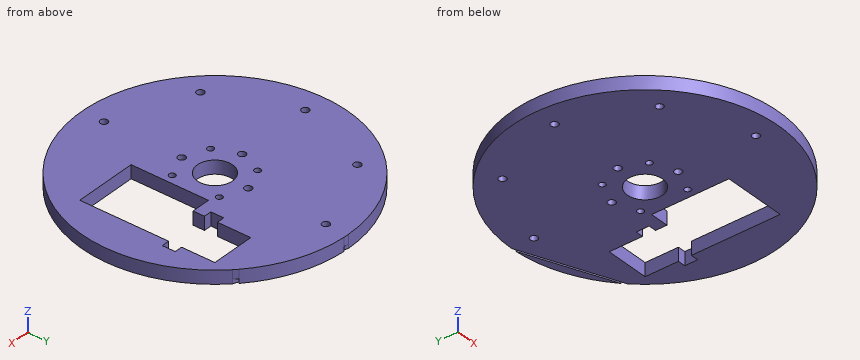
from build123d import *

# Parameters (mm, degrees)
SKETCH1_R              = 60
SKETCH1_R_2            = 8
SKETCH1_R_3            = 1.75
SKETCH1_R_4            = 1.5
BOSS_EXTRUDE1_DEPTH    = 6
CUT_EXTRUDE6_DEPTH     = 86.064681273
CUT_EXTRUDE7_DEPTH     = 2
MOVE_FACE2_OUTLINE_R   = 8
MOVE_FACE2_OUTLINE_R_2 = 7.92
MOVE_FACE2_OUTLINE_R_3 = 1.75
MOVE_FACE2_OUTLINE_R_4 = 1.67
MOVE_FACE2_OUTLINE_R_5 = 1.5
MOVE_FACE2_OUTLINE_R_6 = 1.42
MOVE_FACE2_DEPTH       = 6
MOVE_START             = 2
MOVE_FACE2_2_DEPTH     = 4


# Read off the part's stored shape, not the designer's step: Move Face2
with BuildPart() as part:
    # Sketch1 → Boss-Extrude1 (new body)
    with BuildSketch(Plane.XY):
        Circle(SKETCH1_R)
        Circle(SKETCH1_R_2, mode=Mode.SUBTRACT)
        with Locations((0, -15)):
            Circle(SKETCH1_R_3, mode=Mode.SUBTRACT)
        with Locations((10.606601718, -10.606601718)):
            Circle(SKETCH1_R_4, mode=Mode.SUBTRACT)
        with Locations((0, -50)):
            Circle(SKETCH1_R_3, mode=Mode.SUBTRACT)
        with Locations((-15, 0)):
            Circle(SKETCH1_R_3, mode=Mode.SUBTRACT)
        with Locations((-10.606601718, -10.606601718)):
            Circle(SKETCH1_R_4, mode=Mode.SUBTRACT)
        with Locations((0, 15)):
            Circle(SKETCH1_R_3, mode=Mode.SUBTRACT)
        with Locations((-10.606601718, 10.606601718)):
            Circle(SKETCH1_R_4, mode=Mode.SUBTRACT)
        with Locations((10.606601718, 10.606601718)):
            Circle(SKETCH1_R_4, mode=Mode.SUBTRACT)
        with Locations((-35.355339059, -35.355339059)):
            Circle(SKETCH1_R_3, mode=Mode.SUBTRACT)
        with Locations((-35.355339059, 35.355339059)):
            Circle(SKETCH1_R_3, mode=Mode.SUBTRACT)
        with Locations((-50, 0)):
            Circle(SKETCH1_R_3, mode=Mode.SUBTRACT)
        with Locations((0, 50)):
            Circle(SKETCH1_R_3, mode=Mode.SUBTRACT)
    extrude(amount=BOSS_EXTRUDE1_DEPTH)

    # Sketch7 → Cut-Extrude6 (cut, through all)
    with BuildSketch(Plane(origin=(0, 0, 0), x_dir=(-1, 0, 0), z_dir=(0, 0, -1))):
        Polygon((-43, -26), (-23, -26), (-14.5, -26), (-14.5, 9), (-23, 9), (-23, 14), (-19.5, 14), (-19.5, 20), (-23, 20), (-23, 35), (-43, 35), (-43, 20), (-46.5, 20), (-46.5, 14), (-43, 14), align=None)
    extrude(amount=-CUT_EXTRUDE6_DEPTH, mode=Mode.SUBTRACT)

    # Sketch8 → Cut-Extrude7 (cut)
    with BuildSketch(Plane(origin=(0, 0, 0), x_dir=(-1, 0, 0), z_dir=(0, 0, -1))):
        Polygon((-42.426406871, 42.426406871), (0, 60), (-0.316144007, 60.951441065), (-42.742550878, 43.377847936), align=None)
    extrude(amount=-CUT_EXTRUDE7_DEPTH, mode=Mode.SUBTRACT)

    # Move Face2 outline → Move Face2 (add)
    # profile 1 of 16: a face of its own
    with BuildSketch(Plane.XY):
        with BuildLine():
            ThreePointArc((0.01591808, 60.079997891), (-22.991620616, -55.506682313), (42.47171814, 42.494229705))
            Line((42.47171814, 42.494229705), (0.01591808, 60.079997891))
        make_face()
        with BuildLine():
            Line((0, 60), (42.426406871, 42.426406871))
            ThreePointArc((42.426406871, 42.426406871), (-22.961005942, -55.432771951), (0, 60))
        make_face(mode=Mode.SUBTRACT)
    # profile 2 of 16: a face of its own
    with BuildSketch(Plane.XY):
        with BuildLine():
            ThreePointArc((40.811514416, 44.091118052), (22.991620617, 55.506682313), (2.319029971, 60.035227159))
            Line((2.319029971, 60.035227159), (40.811514416, 44.091118052))
        make_face()
        with BuildLine():
            ThreePointArc((2.767270729, 59.936151134), (22.961005942, 55.432771951), (40.424503007, 44.338014803))
            Line((40.424503007, 44.338014803), (2.767270729, 59.936151134))
        make_face(mode=Mode.SUBTRACT)
    # profile 3 of 16: a face of its own
    with BuildSketch(Plane.XY):
        Circle(MOVE_FACE2_OUTLINE_R)
        Circle(MOVE_FACE2_OUTLINE_R_2, mode=Mode.SUBTRACT)
    # profile 4 of 16: a face of its own
    with BuildSketch(Plane.XY):
        with Locations((0, -15)):
            Circle(MOVE_FACE2_OUTLINE_R_3)
        with Locations((0, -15)):
            Circle(MOVE_FACE2_OUTLINE_R_4, mode=Mode.SUBTRACT)
    # profile 5 of 16: a face of its own
    with BuildSketch(Plane.XY):
        with Locations((10.606601718, -10.606601718)):
            Circle(MOVE_FACE2_OUTLINE_R_5)
        with Locations((10.606601718, -10.606601718)):
            Circle(MOVE_FACE2_OUTLINE_R_6, mode=Mode.SUBTRACT)
    # profile 6 of 16: a face of its own
    with BuildSketch(Plane.XY):
        with Locations((0, -50)):
            Circle(MOVE_FACE2_OUTLINE_R_3)
        with Locations((0, -50)):
            Circle(MOVE_FACE2_OUTLINE_R_4, mode=Mode.SUBTRACT)
    # profile 7 of 16: a face of its own
    with BuildSketch(Plane.XY):
        with Locations((-35.355339059, -35.355339059)):
            Circle(MOVE_FACE2_OUTLINE_R_3)
        with Locations((-35.355339059, -35.355339059)):
            Circle(MOVE_FACE2_OUTLINE_R_4, mode=Mode.SUBTRACT)
    # profile 8 of 16: a face of its own
    with BuildSketch(Plane.XY):
        with Locations((-15, 0)):
            Circle(MOVE_FACE2_OUTLINE_R_3)
        with Locations((-15, 0)):
            Circle(MOVE_FACE2_OUTLINE_R_4, mode=Mode.SUBTRACT)
    # profile 9 of 16: a face of its own
    with BuildSketch(Plane.XY):
        with Locations((-10.606601718, -10.606601718)):
            Circle(MOVE_FACE2_OUTLINE_R_5)
        with Locations((-10.606601718, -10.606601718)):
            Circle(MOVE_FACE2_OUTLINE_R_6, mode=Mode.SUBTRACT)
    # profile 10 of 16: a face of its own
    with BuildSketch(Plane.XY):
        with Locations((0, 15)):
            Circle(MOVE_FACE2_OUTLINE_R_3)
        with Locations((0, 15)):
            Circle(MOVE_FACE2_OUTLINE_R_4, mode=Mode.SUBTRACT)
    # profile 11 of 16: a face of its own
    with BuildSketch(Plane.XY):
        with Locations((-10.606601718, 10.606601718)):
            Circle(MOVE_FACE2_OUTLINE_R_5)
        with Locations((-10.606601718, 10.606601718)):
            Circle(MOVE_FACE2_OUTLINE_R_6, mode=Mode.SUBTRACT)
    # profile 12 of 16: a face of its own
    with BuildSketch(Plane.XY):
        with Locations((10.606601718, 10.606601718)):
            Circle(MOVE_FACE2_OUTLINE_R_5)
        with Locations((10.606601718, 10.606601718)):
            Circle(MOVE_FACE2_OUTLINE_R_6, mode=Mode.SUBTRACT)
    # profile 13 of 16: a face of its own
    with BuildSketch(Plane.XY):
        with Locations((-50, 0)):
            Circle(MOVE_FACE2_OUTLINE_R_3)
        with Locations((-50, 0)):
            Circle(MOVE_FACE2_OUTLINE_R_4, mode=Mode.SUBTRACT)
    # profile 14 of 16: a face of its own
    with BuildSketch(Plane.XY):
        with Locations((-35.355339059, 35.355339059)):
            Circle(MOVE_FACE2_OUTLINE_R_3)
        with Locations((-35.355339059, 35.355339059)):
            Circle(MOVE_FACE2_OUTLINE_R_4, mode=Mode.SUBTRACT)
    # profile 15 of 16: a face of its own
    with BuildSketch(Plane.XY):
        with Locations((0, 50)):
            Circle(MOVE_FACE2_OUTLINE_R_3)
        with Locations((0, 50)):
            Circle(MOVE_FACE2_OUTLINE_R_4, mode=Mode.SUBTRACT)
    # profile 16 of 16: a face of its own
    with BuildSketch(Plane.XY):
        Polygon((14.5, -26), (43, -26), (43, 14), (46.5, 14), (46.5, 20), (43, 20), (43, 35), (23, 35), (23, 20), (19.5, 20), (19.5, 14), (23, 14), (23, 9), (14.5, 9), align=None)
        Polygon((42.92, 14.08), (42.92, -25.92), (14.58, -25.92), (14.58, 8.92), (23.08, 8.92), (23.08, 14.08), (19.58, 14.08), (19.58, 19.92), (23.08, 19.92), (23.08, 34.92), (42.92, 34.92), (42.92, 19.92), (46.42, 19.92), (46.42, 14.08), align=None, mode=Mode.SUBTRACT)
    extrude(amount=MOVE_FACE2_DEPTH)

    # Move Face2 2 outline → Move Face2 2 (add)
    with BuildSketch(Plane.XY.offset(MOVE_START)):
        with BuildLine():
            Line((42.277699454, 42.574594876), (42.47171814, 42.494229705))
            ThreePointArc((42.47171814, 42.494229705), (41.649270334, 43.300631412), (40.811514416, 44.091118052))
            Line((40.811514416, 44.091118052), (40.597304781, 44.179846588))
            ThreePointArc((40.597304781, 44.179846588), (41.44527464, 43.385357092), (42.277699454, 42.574594876))
        make_face()
        with BuildLine():
            ThreePointArc((2.319029971, 60.035227159), (1.167688616, 60.068651585), (0.01591808, 60.079997891))
            Line((0.01591808, 60.079997891), (0.209936765, 59.99963272))
            ThreePointArc((0.209936765, 59.99963272), (1.371845458, 59.98431495), (2.533239607, 59.946498622))
            Line((2.533239607, 59.946498622), (2.319029971, 60.035227159))
        make_face()
    extrude(amount=MOVE_FACE2_2_DEPTH)


solid = part.part
Could you check a few things on this model? Use its own coordinates, in mm. Coordinates: 2 decimals unless noted, no trailing zeros. Order: outer loops, then holes, each group sorted by start corner. A loop starts at its lowest first (then second) coordinate and runs counter-clockwise, first axis right, second up.
Q1. Suppose I cut it at C-C on z = 4.1. Give the number of separate pieces and of enclosed holes in the cut face, and give its area (3 significant figures).
Q2. Suppose I cut it at A-A on y = 0. Please give me the cut outline in (x, z), and give its area (3 significant figures).
Q3. Suppose I cut it at B-B on x = -50. Please give me the cut outline in (y, z).
Q4. Will these pins go through, and if not, where does the flat tip stop? pin 1 (1.5 mm diameter, centred on x = -2.5, z = 4.5, fed in from +Y); pin 2 (1.8 mm diameter, centred on x = 28, z = 4, fed in from -Y); pin 3 (3 mm diameter, centred on x = 20.5, z = 3, fed in from -Y).
Q5. Suppose I cut it at D-D on y = 29.5. Please give me the cut outline in (x, z), and give its area (3 significant figures).
Q6. Please list where these lines run through material, in increasing order: L1, parallel to Y at x = 0, z = 2.2; L2, parallel to X at y = -13.5, z = 3.5; L3, parallel to X at y = 16, z = 2.9.
Answer:
1. separate pieces: 1
1. enclosed holes: 14
1. area: 9,500 mm2
2. outline: (-60.08, 0) - (-51.67, 0) - (-51.67, 6) - (-60.08, 6) - close; (-48.33, 0) - (-16.67, 0) - (-16.67, 6) - (-48.33, 6) - close; (-13.33, 0) - (-7.92, 0) - (-7.92, 6) - (-13.33, 6) - close; (7.92, 0) - (14.58, 0) - (14.58, 6) - (7.92, 6) - close; (42.92, 0) - (60.08, 0) - (60.08, 6) - (42.92, 6) - close
2. area: 416 mm2
3. outline: (-33.31, 0) - (-1.67, 0) - (-1.67, 6) - (-33.31, 6) - close; (1.67, 0) - (33.31, 0) - (33.31, 6) - (1.67, 6) - close
4. pin 1: stops at y = 60.05
4. pin 2: stops at y = -53.62
4. pin 3: stops at y = -57
5. outline: (-52.34, 0) - (23.08, 0) - (23.08, 6) - (-52.34, 6) - close; (42.92, 0) - (52.34, 0) - (52.34, 6) - (42.92, 6) - close
5. area: 509 mm2
6. L1: y = -60.08 to -51.67, -48.33 to -16.67, -13.33 to -7.92, 7.92 to 13.33, 16.67 to 48.33, 51.67 to 60.08
6. L2: x = -58.54 to -0.73, 0.73 to 14.58, 42.92 to 58.54
6. L3: x = -57.91 to -1.34, 1.34 to 19.58, 46.42 to 57.91
